Can you work these out from the model? Positions are in its coordinate system, mm. A direction names the side the tool comes from. Round coordinates to 2 decimals unless told otherwise and drop trailing zeros. Loops run counter-clockwise (first coordinate to the right, second up) from the corner with the lowest first, then second, coordinate; pieces in that order, holes last. Notation, with made-up numbers: M 33.5,-31.75 L 86.5,-31.75 A25 ccw 86.5,-11.75 Z; hole C 79,63 d11. An arc over 180 degrees is marked long. Return JSON: item names as keys, results as strings.
```python
from build123d import *

# Parameters (mm, degrees)
SKETCH_1_W          = 45
SKETCH_1_H          = 15
EXTRUDE_1_DEPTH     = 10
SKETCH_2_W          = 1.6
SKETCH_2_H          = 15
EXTRUDE_2_DEPTH     = 10
SKETCH_3_W          = 8
SKETCH_3_H          = 15
EXTRUDE_3_DEPTH     = 2.5
SKETCH_4_R          = 3.9
EXTRUDE_4_DEPTH     = 0.7
SKETCH_6_R          = 3.5
EXTRUDE_5_DEPTH     = 4
CUT_EXTRUDE_START   = -1
CUT_EXTRUDE_1_DEPTH = 1
SKETCH_8_R          = 0.85
EXTRUDE_6_DEPTH     = 2.5
SKETCH_9_W          = 28.344633457
SKETCH_9_H          = 24.026198997
CUT_EXTRUDE_2_DEPTH = 21.7


with BuildPart() as part:
    # Эскиз1 → Вытянуть1 (new body)
    with BuildSketch(Plane.XY):
        Rectangle(SKETCH_1_W, SKETCH_1_H)
    extrude(amount=EXTRUDE_1_DEPTH)

    # Эскиз2 → Вытянуть2 (add)
    with BuildSketch(Plane.XY.offset(10)):
        with Locations((-21.7, 0)):
            Rectangle(SKETCH_2_W, SKETCH_2_H)
        with Locations((-10.85, 0)):
            Rectangle(SKETCH_2_W, SKETCH_2_H)
        Rectangle(SKETCH_2_W, SKETCH_2_H)
        with Locations((10.85, 0)):
            Rectangle(SKETCH_2_W, SKETCH_2_H)
        with Locations((21.7, 0)):
            Rectangle(SKETCH_2_W, SKETCH_2_H)
    extrude(amount=EXTRUDE_2_DEPTH)

    # Эскиз3 → Вытянуть3 (add)
    with BuildSketch(Plane.XY.offset(10)):
        with Locations((-16.275, 0)):
            Rectangle(SKETCH_3_W, SKETCH_3_H)
        with Locations((-5.425, 0)):
            Rectangle(SKETCH_3_W, SKETCH_3_H)
        with Locations((5.425, 0)):
            Rectangle(SKETCH_3_W, SKETCH_3_H)
        with Locations((16.275, 0)):
            Rectangle(SKETCH_3_W, SKETCH_3_H)
    extrude(amount=EXTRUDE_3_DEPTH)

    # Эскиз4 → Вытянуть4 (add)
    with BuildSketch(Plane.XY.offset(12.5)):
        with Locations(Location((-16.275, 0, 0), (0, 0, 180))):
            Circle(SKETCH_4_R)
        with Locations(Location((-5.425, 0, 0), (0, 0, 180))):
            Circle(SKETCH_4_R)
        with Locations(Location((5.425, 0, 0), (0, 0, 180))):
            Circle(SKETCH_4_R)
        with Locations(Location((16.275, 0, 0), (0, 0, 180))):
            Circle(SKETCH_4_R)
    extrude(amount=EXTRUDE_4_DEPTH)

    # Эскиз6 → Вытянуть5 (add)
    with BuildSketch(Plane.XY.offset(13.2)):
        with Locations((-16.275, 0)):
            Circle(SKETCH_6_R)
        with Locations((-5.425, 0)):
            Circle(SKETCH_6_R)
        with Locations((5.425, 0)):
            Circle(SKETCH_6_R)
        with Locations((16.275, 0)):
            Circle(SKETCH_6_R)
    extrude(amount=EXTRUDE_5_DEPTH)

    # Эскиз7 → Вырез-Вытянуть1 (cut)
    with BuildSketch(Plane.XY.offset(17.2).offset(CUT_EXTRUDE_START)):
        with BuildLine():
            Line((-14.510977508, 3.02294966), (-18.956438169, -2.24941978))
            ThreePointArc((-18.956438169, -2.24941978), (-18.531128818, -2.675795724), (-18.039022492, -3.02294966))
            Line((-18.039022492, -3.02294966), (-13.593561831, 2.24941978))
            ThreePointArc((-13.593561831, 2.24941978), (-14.018871182, 2.675795724), (-14.510977508, 3.02294966))
        make_face()
        with BuildLine():
            Line((-3.660977508, 3.02294966), (-8.106438169, -2.24941978))
            ThreePointArc((-8.106438169, -2.24941978), (-7.681128818, -2.675795724), (-7.189022492, -3.02294966))
            Line((-7.189022492, -3.02294966), (-2.743561831, 2.24941978))
            ThreePointArc((-2.743561831, 2.24941978), (-3.168871182, 2.675795724), (-3.660977508, 3.02294966))
        make_face()
        with BuildLine():
            Line((7.189022492, 3.02294966), (2.743561831, -2.24941978))
            ThreePointArc((2.743561831, -2.24941978), (3.168871182, -2.675795724), (3.660977508, -3.02294966))
            Line((3.660977508, -3.02294966), (8.106438169, 2.24941978))
            ThreePointArc((8.106438169, 2.24941978), (7.681128818, 2.675795724), (7.189022492, 3.02294966))
        make_face()
        with BuildLine():
            Line((18.039022492, 3.02294966), (13.593561831, -2.24941978))
            ThreePointArc((13.593561831, -2.24941978), (14.018871182, -2.675795724), (14.510977508, -3.02294966))
            Line((14.510977508, -3.02294966), (18.956438169, 2.24941978))
            ThreePointArc((18.956438169, 2.24941978), (18.531128818, 2.675795724), (18.039022492, 3.02294966))
        make_face()
    extrude(amount=CUT_EXTRUDE_1_DEPTH, mode=Mode.SUBTRACT)

    # Эскиз8 → Вытянуть6 (add)
    with BuildSketch(Plane(origin=(0, 0, 0), x_dir=(-1, 0, 0), z_dir=(0, 0, -1))):
        with Locations((-5, 0)):
            Circle(SKETCH_8_R)
        with Locations((5, 0)):
            Circle(SKETCH_8_R)
        with Locations((15, 0)):
            Circle(SKETCH_8_R)
        with Locations((-15, 0)):
            Circle(SKETCH_8_R)
    extrude(amount=EXTRUDE_6_DEPTH)

    # Эскиз9 → Вырез-Вытянуть2 (cut)
    with BuildSketch(Plane(origin=(22.5, 0, 0), x_dir=(0, 0, -1), z_dir=(1, 0, 0))):
        with Locations((-8.887417233, 0.294438713)):
            Rectangle(SKETCH_9_W, SKETCH_9_H)
    extrude(amount=-CUT_EXTRUDE_2_DEPTH, mode=Mode.SUBTRACT)


solid = part.part
```
Q1. If I drill on line 1 along X through (y, z) = (-2.5, 10.25) (3 decimals); line 2 along X through (y, z) = (-0.5, 18.25); line 3 along Z through (x, y) = (-13, -5.75), over which ranges is the centre line in solid material (lowest first)?
Results:
{"line 1": "x = -22.5 to -20.9, -20.275 to -12.275, -11.65 to -10.05, -9.425 to -1.425, -0.8 to 0.8", "line 2": "x = -22.5 to -20.9, -11.65 to -10.05, -0.8 to 0.8", "line 3": "z = 0 to 12.5"}
Q2. Suppose I cut it at D-D, the plane x = -11. Please give me the cut outline in (y, z).
Results:
{"outline": "M -7.5,0 L 7.5,0 L 7.5,20 L -7.5,20 Z"}
Q3. On a 3-axis mill with a long thin cutter (end or side, diameter ignored), from which of +Z, -Z, +X, -X, +Y, -Y can I reach the whole of each face in a straight line? I mean faces 1 (the flat face through (-7, 1, 17.2)), 2 (the flat face through (-15.847, -0.424, 16.693)), 3 (the flat face through (-11, 0, 20)). Say none if no direction works.
Results:
{"face 1": "+Z, +Y, -Y", "face 2": "+Z", "face 3": "+Z, +X, -X, +Y, -Y"}
Q4. Suppose I cut it at A-A, the plane y = 5.5. Please give me the cut outline in (x, z) (3 decimals).
Results:
{"outline": "M -22.5,0 L 0.8,0 L 0.8,20 L -0.8,20 L -0.8,10 L -1.425,10 L -1.425,12.5 L -9.425,12.5 L -9.425,10 L -10.05,10 L -10.05,20 L -11.65,20 L -11.65,10 L -12.275,10 L -12.275,12.5 L -20.275,12.5 L -20.275,10 L -20.9,10 L -20.9,20 L -22.5,20 Z"}
Q5. Suppose I cut it at B-B, the plane x = -5. Please give me the cut outline in (y, z), plus the area to 3 significant figures.
Results:
{"outline": "M -7.5,0 L -0.85,0 L -0.85,-2.5 L 0.85,-2.5 L 0.85,0 L 7.5,0 L 7.5,12.5 L 3.88,12.5 L 3.88,13.2 L 3.47,13.2 L 3.47,17.2 L 1.43,17.2 L 1.43,16.2 L -0.43,16.2 L -0.43,17.2 L -3.47,17.2 L -3.47,13.2 L -3.88,13.2 L -3.88,12.5 L -7.5,12.5 Z", "area": "223 mm2"}
Q6. Thinking about a two-plate mould opening in X: for faces 4 (the flat face through (-22.5, 0, 10)), 5 (the flat face through (-5, 0, -2.5)), 6 (the cylindrical face through (-15.785, -0.326, -1.232)), which applies, pulls with the +X half, pulls with the -X half, needs draft (parallel to the pull), parting line crosses it, or undercut?
Results:
{"face 4": "pulls with the -X half", "face 5": "needs draft", "face 6": "undercut"}
Q7. I'm going to push flat-ended pins straight in: pin 1 Ø4 at (x, y) = (-15, 0.5) entering from +Z; pin 2 Ø0.7 at (x, y) = (-9.5, 3.5) entering from +Z. Where does each tip first touch, or does it pass through?
Results:
{"pin 1": "stops at z = 17.2", "pin 2": "stops at z = 12.5"}
Q8. Suppose I cut it at C-C, the plane x = -8.5. Please give me the cut outline in (y, z).
Results:
{"outline": "M -7.5,0 L 7.5,0 L 7.5,12.5 L 2.4,12.5 L 2.4,13.2 L 1.67,13.2 L 1.67,17.2 L -1.67,17.2 L -1.67,13.2 L -2.4,13.2 L -2.4,12.5 L -7.5,12.5 Z"}
